The model under review builds one solid part; all positions refer to its coordinate system, in mm. A direction names the side the tool comes from. Round coordinates to 2 decimals unless told otherwise and drop trailing zeros. Loops run counter-clockwise (first coordinate to the right, second up) from the corner with the lowest first, then second, coordinate; pieces in that order, holes last. Notation, with made-up numbers: (45, -16) -> (100, -16) arc R25 cw to (100, 21) -> close; hole circle Ø8 at (-12.5, 25). An arc over 180 degrees is marked (long way). Write each question's results on one line, items separated by ' | '. Start each with the question number.
Item 1: For L1, parallel to Z at x = 8.5, y = 15.5; L2, parallel to Y at x = -12.5, z = 109; L3, parallel to Z at x = 16.5, y = -29, list the stretches that pass through material, from the lowest coordinate up. Write a range as from..to.
Item 2: Clearance check with flat-ended pins moving along their axes: pin 1 Ø1 at (x, z) = (-11, 36) entering from +Y; pin 2 Ø3.5 at (x, y) = (12.5, 0) entering from -Z; pin 3 Ø1.6 at (y, z) = (-29.5, 69) entering from -X. State where each tip first meets the part, or that it passes through.
Item 3: We need section B-B (y = 9.5). Give the boundary of the cut face in (x, z).
Item 4: Tool access review of faces 1 (the cylindrical face through (-20.68, -29.48, 67.1)), 2 (the flat face through (-26.08, -5.86, 107.15)), 3 (the flat face through (-1, -4, 106)): name each direction out of +Z, -Z, +X, -X, +Y, -Y from which nothing blocks a thin tool from reaching the whole face with its end or side.
Item 5: We need section C-C (x = -12.5). Give the boundary of the cut face in (y, z).
Item 6: We need section A-A (x = 0). Give the number of separate pieces and of enclosed holes in the cut face, and give its area (3 significant figures).
Item 7: We need section D-D (y = -14). Give the boundary of the cut face in (x, z), and give its area (3 significant figures).
Item 8: Mouldability with a two-part tool opening along Y and no side actions: class faces 4 (the cylindrical face through (11, 0, 108)), 5 (the flat face through (25, -6, 1)), 6 (the cylindrical face through (-0.35, -27.43, 3.6)) as pulls with the +Y half, pulls with the -Y half, needs draft (parallel to the pull), parting line crosses it, or undercut.
from build123d import *

# Parameters (mm, degrees)
SKETCH_1_W      = 50
SKETCH_1_H      = 51
SKETCH_1_R      = 6
SKETCH_1_R_2    = 3
EXTRUDE_1_DEPTH = 3
SKETCH_2_W      = 16
SKETCH_2_H      = 6
EXTRUDE_2_DEPTH = 3
SKETCH_3_W      = 49
SKETCH_3_H      = 51
SKETCH_3_R      = 1.5
EXTRUDE_3_DEPTH = 4
FILLET_2_R      = 2
FILLET_3_R      = 2
FILLET_4_R      = 2
FILLET_5_R      = 2
FILLET_6_R      = 2
EXTRUDE_5_DEPTH = 51


with BuildPart() as part:
    # 草图1 → 凸台-拉伸1 (new body)
    with BuildSketch(Plane.XY):
        with Locations((0, -5.5)):
            Rectangle(SKETCH_1_W, SKETCH_1_H)
        Circle(SKETCH_1_R, mode=Mode.SUBTRACT)
        with Locations((12.5, 0)):
            Circle(SKETCH_1_R_2, mode=Mode.SUBTRACT)
        with Locations((-12.5, 0)):
            Circle(SKETCH_1_R_2, mode=Mode.SUBTRACT)
        with Locations((0, 9.5)):
            Circle(SKETCH_1_R_2, mode=Mode.SUBTRACT)
        with Locations((0, -9.5)):
            Circle(SKETCH_1_R_2, mode=Mode.SUBTRACT)
    extrude(amount=EXTRUDE_1_DEPTH)

    # 草图2 → 凸台-拉伸2 (add)
    with BuildSketch(Plane.XZ.offset(31)):
        Polygon((-25, 3), (-25, 106), (24, 106), (25, 3), align=None)
        with Locations((-13.25, 39.5)):
            Rectangle(SKETCH_2_W, SKETCH_2_H, mode=Mode.SUBTRACT)
        Polygon((4.866266466, 42.54910809), (4.92451752, 36.549390862), (20.923763461, 36.704727007), (20.865512407, 42.704444235), align=None, mode=Mode.SUBTRACT)
        with Locations((-13.25, 69.5)):
            Rectangle(SKETCH_2_W, SKETCH_2_H, mode=Mode.SUBTRACT)
        Polygon((20.865512407, 66.295555765), (20.923763461, 72.295272993), (4.92451752, 72.450609138), (4.866266466, 66.45089191), align=None, mode=Mode.SUBTRACT)
    extrude(amount=-EXTRUDE_2_DEPTH)

    # 草图3 → 凸台-拉伸3 (add)
    with BuildSketch(Plane.XY.offset(106)):
        with Locations((-0.5, -5.5)):
            Rectangle(SKETCH_3_W, SKETCH_3_H)
        with Locations((-12.5, 0)):
            Circle(SKETCH_3_R, mode=Mode.SUBTRACT)
        with Locations((12.5, 0)):
            Circle(SKETCH_3_R, mode=Mode.SUBTRACT)
        with Locations((0, -9.5)):
            Circle(SKETCH_3_R, mode=Mode.SUBTRACT)
        with Locations((0, 9.5)):
            Circle(SKETCH_3_R, mode=Mode.SUBTRACT)
        with Locations((0, 13.75)):
            Circle(SKETCH_3_R, mode=Mode.SUBTRACT)
    extrude(amount=EXTRUDE_3_DEPTH)

    # 圆角2
    fillet_2_edges = [part.edges().sort_by_distance(p)[0] for p in [
        (-5.25, -29.5, 36.5),
    ]]
    fillet(fillet_2_edges, radius=FILLET_2_R)

    # 圆角3
    fillet_3_edges = [part.edges().sort_by_distance(p)[0] for p in [
        (-21.25, -29.5, 36.5),
        (-21.25, -29.5, 42.5),
        (-5.25, -29.5, 42.5),
    ]]
    fillet(fillet_3_edges, radius=FILLET_3_R)

    # 圆角4
    fillet_4_edges = [part.edges().sort_by_distance(p)[0] for p in [
        (20.865512407, -29.5, 42.704444235),
        (20.923763461, -29.5, 36.704727007),
        (4.92451752, -29.5, 36.549390862),
        (4.866266466, -29.5, 42.54910809),
        (-21.25, -29.5, 66.5),
        (-21.25, -29.5, 72.5),
        (-5.25, -29.5, 72.5),
        (-5.25, -29.5, 66.5),
        (4.866266466, -29.5, 66.45089191),
        (4.92451752, -29.5, 72.450609138),
        (20.923763461, -29.5, 72.295272993),
        (20.865512407, -29.5, 66.295555765),
    ]]
    fillet(fillet_4_edges, radius=FILLET_4_R)

    # 圆角5
    fillet_5_edges = [part.edges().sort_by_distance(p)[0] for p in [
        (0, -28, 3),
    ]]
    fillet(fillet_5_edges, radius=FILLET_5_R)

    # 圆角6
    fillet_6_edges = [part.edges().sort_by_distance(p)[0] for p in [
        (0, -31, 0),
    ]]
    fillet(fillet_6_edges, radius=FILLET_6_R)

    # 草图6 → 凸台-拉伸5 (add)
    with BuildSketch(Plane(origin=(0, -31, 0), x_dir=(-1, 0, 0), z_dir=(0, -1, 0))):
        Polygon((-24, -108.9), (-23.989320388, -107.1), (-26.2, -107.2), (-26.2, -108.8), align=None)
        Polygon((25, -108.9), (24.989320388, -107.1), (27.2, -107.2), (27.2, -108.8), align=None)
    extrude(amount=-EXTRUDE_5_DEPTH)


solid = part.part
Here are the results:
1) L1: z = 0..3, 106..110 | L2: y = -31..-1.5, 1.5..20 | L3: z = 0..36.66, 42.66..66.34, 72.34..110
2) pin 1: stops at y = -28 | pin 2: stops at z = 106 | pin 3: stops at x = -25
3) outline: (-27.2, 107.2) -> (-25, 107.1) -> (-25, 106) -> (-1.5, 106) -> (-1.5, 110) -> (-25, 110) -> (-25, 108.9) -> (-27.2, 108.8) -> close; (-25, 0) -> (-3, 0) -> (-3, 3) -> (-25, 3) -> close; (1.5, 106) -> (24, 106) -> (24, 107.1) -> (26.2, 107.2) -> (26.2, 108.8) -> (24, 108.9) -> (24, 110) -> (1.5, 110) -> close; (3, 0) -> (25, 0) -> (25, 3) -> (3, 3) -> close
4) face 1: +Y, -Y | face 2: -Z, -X, +Y, -Y | face 3: +X, -X, +Y
5) outline: (-31, 2) arc R2 ccw to (-29, 0) -> (-3, 0) -> (-3, 3) -> (-26, 3) arc R2 cw to (-28, 5) -> (-28, 36.5) -> (-31, 36.5) -> close; (-31, 42.5) -> (-28, 42.5) -> (-28, 66.5) -> (-31, 66.5) -> close; (-31, 72.5) -> (-28, 72.5) -> (-28, 106) -> (-1.5, 106) -> (-1.5, 110) -> (-31, 110) -> close; (1.5, 106) -> (20, 106) -> (20, 110) -> (1.5, 110) -> close; (3, 0) -> (20, 0) -> (20, 3) -> (3, 3) -> close
6) separate pieces: 7 | enclosed holes: 0 | area: 558 mm2
7) outline: (-27.2, 107.2) -> (-25, 107.1) -> (-25, 106) -> (24, 106) -> (24, 107.1) -> (26.2, 107.2) -> (26.2, 108.8) -> (24, 108.9) -> (24, 110) -> (-25, 110) -> (-25, 108.9) -> (-27.2, 108.8) -> close; (-25, 0) -> (25, 0) -> (25, 3) -> (-25, 3) -> close | area: 353 mm2
8) face 4: undercut | face 5: needs draft | face 6: pulls with the +Y half
